from build123d import *

# Parameters (mm, degrees)
F0_W     = 30.48
F0_H     = 5.08
F0_R     = 3.175
F1_DEPTH = 6.35
F2_DEPTH = 6.35


with BuildPart() as f1:
    # F0 (on Top) → F1 (new body)
    with BuildSketch(Plane.XY):
        with BuildLine():
            Line((38.1, -25.4), (38.1, 25.4))
            Line((38.1, 25.4), (-38.1, 25.4))
            Line((-38.1, 25.4), (-38.1, 9.525))
            ThreePointArc((-38.1, 9.525), (-31.3648079092, 6.7351920908), (-28.575, 0))
            ThreePointArc((-28.575, 0), (-31.3648079092, -6.7351920908), (-38.1, -9.525))
            Line((-38.1, -9.525), (-38.1, -25.4))
            Line((-38.1, -25.4), (38.1, -25.4))
        make_face()
        with Locations((16.51, -13.97)):
            Rectangle(F0_W, F0_H, mode=Mode.SUBTRACT)
        with Locations((16.51, 13.97)):
            Rectangle(F0_W, F0_H, mode=Mode.SUBTRACT)
        with BuildLine():
            Line((-38.1, 9.525), (-38.1, 25.4))
            Line((-38.1, 25.4), (-69.85, 25.4))
            ThreePointArc((-69.85, 25.4), (-74.3401280605, 23.5401280605), (-76.2, 19.05))
            Line((-76.2, 19.05), (-76.2, -19.05))
            ThreePointArc((-76.2, -19.05), (-74.3401280605, -23.5401280605), (-69.85, -25.4))
            Line((-69.85, -25.4), (-38.1, -25.4))
            Line((-38.1, -25.4), (-38.1, -9.525))
            ThreePointArc((-38.1, -9.525), (-47.625, 0), (-38.1, 9.525))
        make_face()
        with Locations((-57.15, -17.526)):
            Circle(F0_R, mode=Mode.SUBTRACT)
        with Locations((-57.15, 17.526)):
            Circle(F0_R, mode=Mode.SUBTRACT)
    extrude(amount=F1_DEPTH)

    # F2 (add): a face of the model
    f2_faces = [f1.faces().sort_by_distance(p)[0] for p in [
        (-19.4796748363, 0, 6.35),
    ]]
    extrude(f2_faces, amount=-F2_DEPTH)


solid = f1.part
Geometry check sheet. Reference: the model listing, model coordinates, mm. A direction names the side the tool comes from. Round coordinates to 2 decimals unless told otherwise and drop trailing zeros. Loops run counter-clockwise (first coordinate to the right, second up) from the corner with the lowest first, then second, coordinate; pieces in that order, holes last. Notation, with made-up numbers: (70.5, -26.5) - (99.5, -26.5) arc R26 cw to (99.5, -0.5) - close; hole circle Ø2 at (12, 22). An arc over 180 degrees is marked (long way). One line per question, with ' | ' between items. Start each with the question number.
1. Depth check by flat-ended pin: pin 1 (6 mm diameter, centred on x = -34, y = -3, fed in from +Z). Enter the tip coordinate at first touch or a pass-through.
2. Cross-section at B-B on x = -38.1. Record the cut outline in (y, z) (3 decimals), then the cut area to 3 significant figures.
3. Cross-section at D-D on z = 5. Record the cut outline in (x, y) (3 decimals), then the cut area to 3 significant figures.
4. Tool access check on faces 5 (the face through (38.1, 0, 3)), 6 (the face through (1.27, 14, 3)). Record the directions out of +Z, -Z, +X, -X, +Y, -Y that give a thin tool (end or side, any length) a straight path to the whole face; none if there is none.
5. Cross-section at A-A on y = 0. Record the cut outline in (x, z) (3 decimals).
6. Scan lines: line 1 (Y direction, x = -57.15, z = 5); line 2 (Y direction, x = -38.1, z = 3.25) (3 decimals); line 3 (X direction, y = -16, z = 2.5). Record each from-to range of solid material in increasing order. Write a range as [from, to].
7. Cross-section at C-C on x = 17. Record the cut outline in (y, z).
8. Draft check along Y on faces 1 (the face through (-74.39, -23.49, 3.13)), 2 (the face through (16, -16.51, 3)), 3 (the face through (-74.29, 23.59, 3.13)), 4 (the face through (-20, 0, 6.35)). Enter one of: released by +Y, released by -Y, zero draft, split by the parting line, or undercut.
Taken from the geometry:
1) pin 1: through
2) outline: (-25.4, 0) - (-9.525, 0) - (-9.525, 6.35) - (-25.4, 6.35) - close; (9.525, 0) - (25.4, 0) - (25.4, 6.35) - (9.525, 6.35) - close | area: 202 mm²
3) outline: (-76.2, -19.05) arc R6.35 ccw to (-69.85, -25.4) - (38.1, -25.4) - (38.1, 25.4) - (-69.85, 25.4) arc R6.35 ccw to (-76.2, 19.05) - close; hole circle Ø6.35 at (-57.15, -17.526); hole circle Ø6.35 at (-57.15, 17.526); hole circle Ø19.05 at (-38.1, 0); hole (1.27, -16.51) - (31.75, -16.51) - (31.75, -11.43) - (1.27, -11.43) - close; hole (1.27, 11.43) - (31.75, 11.43) - (31.75, 16.51) - (1.27, 16.51) - close | area: 5,130 mm²
4) face 5: +Z, -Z, +X, +Y, -Y | face 6: +Z, -Z
5) outline: (-76.2, 0) - (-47.625, 0) - (-47.625, 6.35) - (-76.2, 6.35) - close; (-28.575, 0) - (38.1, 0) - (38.1, 6.35) - (-28.575, 6.35) - close
6) line 1: [-25.4, -20.7], [-14.35, 14.35], [20.7, 25.4] | line 2: [-25.4, -9.525], [9.525, 25.4] | line 3: [-76.2, -59.93], [-54.37, 1.27], [31.75, 38.1]
7) outline: (-25.4, 0) - (-16.51, 0) - (-16.51, 6.35) - (-25.4, 6.35) - close; (-11.43, 0) - (11.43, 0) - (11.43, 6.35) - (-11.43, 6.35) - close; (16.51, 0) - (25.4, 0) - (25.4, 6.35) - (16.51, 6.35) - close
8) face 1: released by -Y | face 2: undercut | face 3: released by +Y | face 4: zero draft
